Design review of the part shown in the three views and the two pictorial views. Dimensions are in mm from the part's minimum x, y and z. Give positions to 0.01 mm unless a question says otherwise; leave off trailing zeros. Loops run counter-clockwise (first coordinate to the right, second up) from the corner with the lowest first, then second, coordinate; pieces in that order, holes last. Notation, with made-up numbers: M 71.5,88 L 126.5,88 A23 cw 126.5,124 Z; hole C 4.5,-29 d6. An arc over 180 degrees is marked long. Return JSON: item names as keys, results as strings. Group by question number.
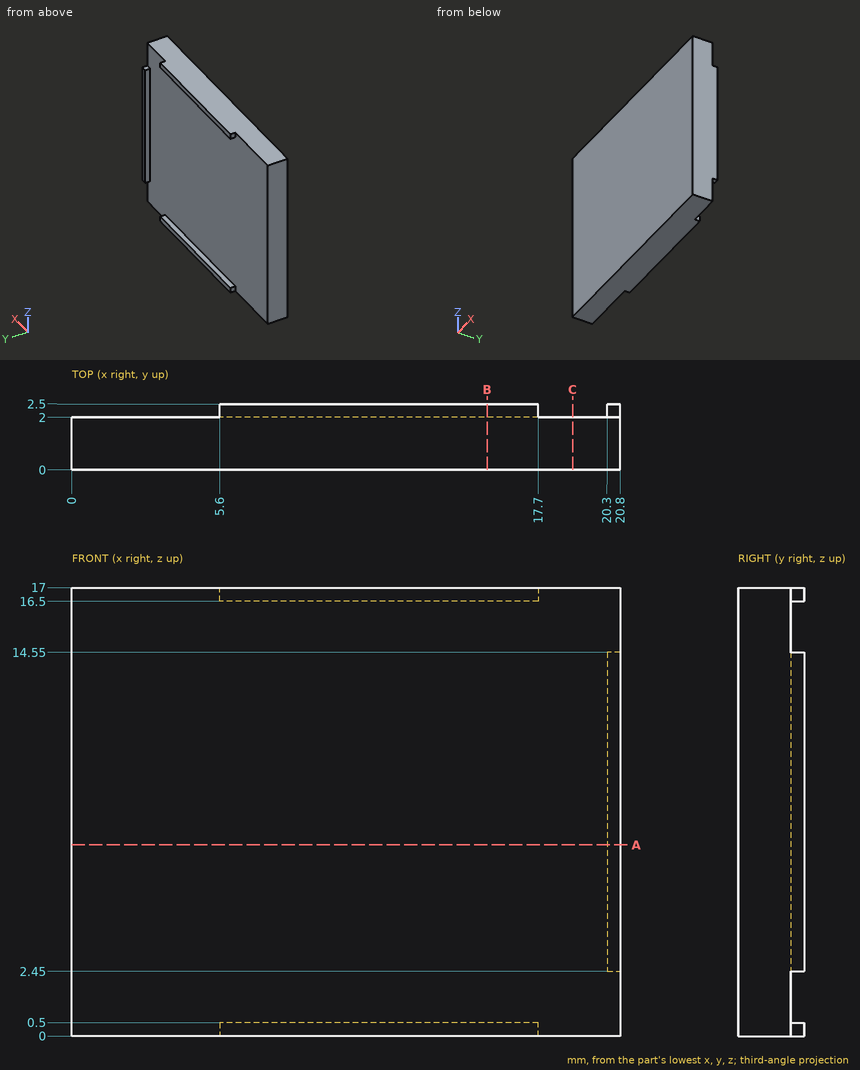
(1) For pin 1 (0.6 mm diameter, centred on y = 2, z = 11, fed in from -X); pin 2 (8.5 mm diameter, centred on x = 13.5, z = 8, fed in from +Y); pin 3 (0.6 mm diameter, centred on y = 2.5, z = 16.5, fed in from -X), all flat-tipped, find the tip position at first contact; note any pin that passes through.
(2) Add section C-C (x = 19). Write out the cut boundary in (y, z).
(3) Add section B-B (x = 15.75). Write out the cut boundary in (y, z), and give its area (3 significant figures).
(4) For probe 1 along Z at (x, y) = (17.5, 2.05); probe 2 along Y at (x, z) = (11.25, 12.75); probe 3 along X at (y, z) = (2.15, 8), list the stretches that pass through material, from the lowest coordinate up.
(5) Add section A-A (z = 7.25). Write out the cut boundary in (x, y).
Verdict:
{
 "1": {"pin 1": "stops at x = 0", "pin 2": "stops at y = 2", "pin 3": "stops at x = 5.6"},
 "2": {"outline": "M 0,0 L 2,0 L 2,17 L 0,17 Z"},
 "3": {"outline": "M 0,0 L 2.5,0 L 2.5,0.5 L 2,0.5 L 2,16.5 L 2.5,16.5 L 2.5,17 L 0,17 Z", "area": "34.5 mm²"},
 "4": {"probe 1": "z = 0 to 0.5, 16.5 to 17", "probe 2": "y = 0 to 2", "probe 3": "x = 20.3 to 20.8"},
 "5": {"outline": "M 0,0 L 20.8,0 L 20.8,2.5 L 20.3,2.5 L 20.3,2 L 0,2 Z"}
}
